Autodesk Inventor part; units mm, degrees
ref_plane "Work Plane1" through (29, 0, 0) normal (0, -1, 0) x (1, 0, 0)
ref_plane "YZ Plane" through (0, 0, 0) normal (1, 0, 0) x (0, 1, 0)
ref_plane "XZ Plane" through (0, 0, 0) normal (0, 1, 0) x (-1, 0, 0)
sketch "Rascunho1" plane through (0, 0, 0) normal (0, 0, 1) x (1, 0, 0)
  line L0 (-2.3333, 0) -> (50, 0)
  line L1 (50, 0) -> (50, 5)
  line L2 (50, 5) -> (15, 5)
  line L3 (15, 5) -> (14.0797, 5)
  line L4 (14.0797, 5) -> (0, 5)
  line L5 (0, 5) -> (0, 8)
  line L6 (0, 8) -> (-10, 8)
  line L7 (-10, 8) -> (-10, 4.6188)
  line L8 (-10, 4.6188) -> (-5, 4.6188)
  line L9 (-5, 4.6188) -> (-2.3333, 0)
  line L10 (-24, 0) -> (74, 0)
  line L11 (0, -1.6) -> (0, 9.6)
  line L12 (15, 5) -> (0, 5) construction
  dimension "d1" = 35
  dimension "d2" = 0.9203
  dimension "d3" = 10
  dimension "d4" = 5
  dimension "d5" = 60
  dimension "d6" = 10
  dimension "d7" = 10
  dimension "d8" = 9.2376
  dimension "d9" = 16
  dimension "d26" = 50
revolve "Corpo" add sketch "Rascunho1" angle 360 about axis through (-2.3333, 0, 0) along (1, 0, 0)
sketch "Rascunho2" plane through (-10, 0, 0) normal (-1, 0, 0) x (0, 0, 1)
  circle A0 centre (0, 0) radius 4.6188
  line L0 (0, -11.2) -> (0, 11.2)
  line L1 (-11.2, 0) -> (11.2, 0)
  line L2 (4.6188, 0) -> (2.3094, -4)
  line L3 (2.3094, -4) -> (-2.3094, -4)
  line L4 (-2.3094, -4) -> (-4.6188, 0)
  line L5 (-4.6188, 0) -> (-2.3094, 4)
  line L6 (-2.3094, 4) -> (2.3094, 4)
  line L7 (2.3094, 4) -> (4.6188, 0)
extrude "Fenda" add sketch "Rascunho2" against normal up to next contours L7 A0 | A0 L2 | L6 L0 A0 | A0 L0 L3 | L0 L6 A0 | A0 L3 L0 | L4 A0 | A0 L5
fillet "Raio de arredondamento1" radius 1 1 edges at (-10, -8, 0)
thread "Rosca"
chamfer "Chanfrar1" distance 0.9202 distance2 0.9202 1 edges at (50, -5, 0) measured on face at (50, -0.8768, -0.3989)
ref_plane "Work Plane1" through (29, 0, 0) normal (0, -1, 0) x (1, 0, 0)
fillet "Fillet2" radius 0.1 1 edges at (0, -5, 0)
equation "\"d1\" = GEL"
equation "\"d3\" = KOH"
equation "\"d4\" = INTI"
equation "\"d6\" = GD"
equation "\"d7\" = BDM"
equation "\"d8\" = 1.1547 * SW"
equation "\"d9\" = KOD"
equation "\"d26\" = NLG"
equation "\"d17\" = RR"
equation "\"d13\" = GEL"
equation "\"d15\" = -0.5 * SPD + 0.5 * GD"
equation "\"d16\" = GUL"
equation "\"d30\" = R"
equation "\"GD\" = NND"
equation "\"NLG\" = 50"
equation "\"GEL\" = 35"
equation "\"KOD\" = 16"
equation "\"KOH\" = 10"
equation "\"INTI\" = 5"
equation "\"GAL\" = 0.61345 * PTC"
equation "\"GUL\" = 0.61345 * PTC"
equation "\"BDM\" = NND"
equation "\"SW\" = 8"
equation "\"RR\" = 0.1 * KOH"
equation "\"SPD\" = NND - 1.2269 * PTC"
equation "\"R\" = 0.1"
equation "\"TOA\" = 30deg"
equation "\"GD1\" = THREADDIA - 1.2269 * PTC"
equation "\"FAWI\" = 45deg"
equation "\"ANG\" = 120deg"
equation "\"PTC\" = 1.5"
equation "\"E0\" = 1.155 * SW"
properties part number "DIN 912 - M10x50" material "Aço Inox AISI 304"
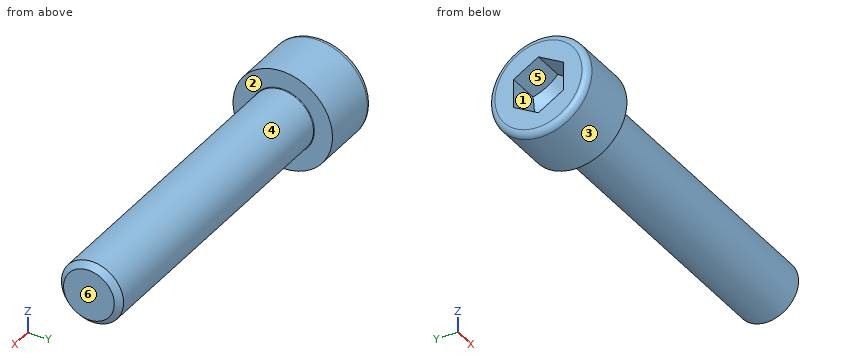
The listing builds one solid part. Answer for the finished solid, in the listing's coordinates (mm). Face numbers are marked on the shaded views. A direction names the side the tool comes from. Coordinates: 2 decimals unless noted, no trailing zeros. Loops run counter-clockwise (first coordinate to the right, second up) from the corner with the lowest first, then second, coordinate; pieces in that order, holes last. Notation, with made-up numbers: (14.5, -23) -> (21.5, -23) arc R29 ccw to (21.5, 13) -> close; hole circle Ø1 at (70.5, -14.5). An arc over 180 degrees is marked (long way). Use one line per item in the form item = value. Start each with the question number.
Item 1: A tool of negligible diameter and unlimited length cuts with its end or side. For the marked faces 1, 2 and 3, from which of +Z, -Z, +X, -X, +Y, -Y can it reach the whole face along a straight path? Write none if from no direction.
Item 2: Flat-ended cylindrical pins translate along their axes: pin 1 Ø1 at (x, y) = (39.5, 1.5) entering from +Z; pin 2 Ø8 at (x, z) = (9, -4.5) entering from -Y; pin 3 Ø4 at (y, z) = (-5.5, 5.5) entering from -X; pin 4 Ø1 at (x, z) = (31.5, -2.5) entering from -Y. Find the tip coordinate at first contact, or state that the pin passes through.
Item 3: The part is cut by section A-A on x = 11.5. Determine the outline of the cut face in (y, z), then the cut area to 3 significant figures.
Item 4: The mould has two halves that part along Z. Classify the marked faces 4, 5 and 6: released by +Z, released by -Z, zero draft, split by the parting line, or undercut.
Item 5: Consider L1, parallel to Z at x = 7, y = 0; L2, parallel to X at y = 5.25, z = -3.5; L3, parallel to Y at x = -6.5, z = 3.5. Determine where each line is inside the solid, lowest interval first. Write a range as [from, to].
Answer key:
q1.face_1 = -X
q1.face_2 = +X
q1.face_3 = +X, -X
q2.pin_1 = 4.9
q2.pin_2 = -4.97
q2.pin_3 = -10
q2.pin_4 = -4.58
q3.outline = circle Ø10 at (0, 0)
q3.area = 78.5 mm2
q4.face_4 = split by the parting line
q4.face_5 = undercut
q4.face_6 = zero draft
q5.L1 = [-5, 5]
q5.L2 = [-10, 0]
q5.L3 = [-7.19, -1.94], [1.94, 7.19]
